Source: CAD feature listing. Evaluate the final solid. Frame: model axes, mm. A direction names the side the tool comes from. Give positions to 0.01 mm unless a question says otherwise; leave off trailing zeros. Write each loop counter-clockwise with the first axis right and the second up, starting at its lowest first coordinate (ties: lowest second). Pieces come first, ordered by that corner, then holes. Notation, with made-up numbers: (25, 42) -> (30, 42) arc R30 ccw to (30, 79) -> close; hole circle Ø11 at (71, -2). An arc over 180 degrees is marked (long way). Answer as a JSON object with one key per item and string values. Group by question number.
Item 1: Section query A-A on y = 7.5. Return the cut outline in (x, z), plus the area to 3 significant figures.
Item 2: Pull-direction query (Y, two-part tool) for faces 1 (the face through (17, 0, 5)), 2 (the face through (19.7, 10, 5)), 3 (the face through (13, 11, 0)); classes: pulls with the +Y half, pulls with the -Y half, needs draft (parallel to the pull), parting line crosses it, or undercut.
Item 3: Ray query, probe 1 along X at (y, z) = (11, 5); probe 2 along Y at (x, z) = (27, 7.5). Return the intervals inside material, ascending. Write a range as from..to.
Item 4: Section query C-C on z = 2.75. Return the cut outline in (x, y), plus the area to 3 significant figures.
Item 5: Access query for faces 4 (the face through (17, 21, 5)), 5 (the face through (27, 16, 5)). Directions: +Z, -Z, +X, -X, +Y, -Y. A direction counts if a zero-diameter tool reaches every point of the face in a straight line with its end or side. Return the directions, or none.
Item 6: Section query B-B on x = 16. Return the cut outline in (y, z), plus the area to 3 significant figures.
from build123d import *

# Parameters (mm, degrees)
BOX002_W     = 4.7
BOX002_H     = 11
BOX002_DEPTH = 10
BOX003_W     = 4.7
BOX003_H     = 11
BOX003_DEPTH = 10
BOX001_W     = 4.7
BOX001_H     = 11
BOX001_DEPTH = 10
BOX_W        = 35
BOX_H        = 21
BOX_DEPTH    = 10


with BuildPart() as cubo002:
    # Box002 → Box002 (new body)
    with BuildSketch(Plane(origin=(15, 5, 0), x_dir=(1, 0, 0), z_dir=(0, 0, 1))):
        with Locations((2.35, 5.5)):
            Rectangle(BOX002_W, BOX002_H)
    extrude(amount=BOX002_DEPTH)


with BuildPart() as cubo003:
    # Box003 → Box003 (new body)
    with BuildSketch(Plane(origin=(25, 5, 0), x_dir=(1, 0, 0), z_dir=(0, 0, 1))):
        with Locations((2.35, 5.5)):
            Rectangle(BOX003_W, BOX003_H)
    extrude(amount=BOX003_DEPTH)


with BuildPart() as cubo001:
    # Box001 → Box001 (new body)
    with BuildSketch(Plane(origin=(5, 5, 0), x_dir=(1, 0, 0), z_dir=(0, 0, 1))):
        with Locations((2.35, 5.5)):
            Rectangle(BOX001_W, BOX001_H)
    extrude(amount=BOX001_DEPTH)


with BuildPart() as cut002:
    # Box → Box (new body)
    with BuildSketch(Plane.XY):
        with Locations((17.5, 10.5)):
            Rectangle(BOX_W, BOX_H)
    extrude(amount=BOX_DEPTH)

    # Cut: cut Cubo001
    add(cubo001.part, mode=Mode.SUBTRACT)

    # Cut001: cut Cubo003
    add(cubo003.part, mode=Mode.SUBTRACT)

    # Cut002: cut Cubo002
    add(cubo002.part, mode=Mode.SUBTRACT)


solid = cut002.part
Worked answers:
{
 "1": {"outline": "(0, 0) -> (5, 0) -> (5, 10) -> (0, 10) -> close; (9.7, 0) -> (15, 0) -> (15, 10) -> (9.7, 10) -> close; (19.7, 0) -> (25, 0) -> (25, 10) -> (19.7, 10) -> close; (29.7, 0) -> (35, 0) -> (35, 10) -> (29.7, 10) -> close", "area": "209 mm^2"},
 "2": {"face 1": "pulls with the -Y half", "face 2": "undercut", "face 3": "needs draft"},
 "3": {"probe 1": "0..5, 9.7..15, 19.7..25, 29.7..35", "probe 2": "0..5, 16..21"},
 "4": {"outline": "(0, 0) -> (35, 0) -> (35, 21) -> (0, 21) -> close; hole (5, 5) -> (9.7, 5) -> (9.7, 16) -> (5, 16) -> close; hole (15, 5) -> (19.7, 5) -> (19.7, 16) -> (15, 16) -> close; hole (25, 5) -> (29.7, 5) -> (29.7, 16) -> (25, 16) -> close", "area": "580 mm^2"},
 "5": {"face 4": "+Z, -Z, +X, -X, +Y", "face 5": "+Z, -Z"},
 "6": {"outline": "(0, 0) -> (5, 0) -> (5, 10) -> (0, 10) -> close; (16, 0) -> (21, 0) -> (21, 10) -> (16, 10) -> close", "area": "100 mm^2"}
}
